The drawing under review shows one solid part. Ordinate dimensions are in mm from its lowest x, y, z. Coordinates: 2 decimals unless noted, no trailing zeros. Loops run counter-clockwise (first coordinate to the right, second up) from the corner with the lowest first, then second, coordinate; pieces in that order, holes last. Notation, with made-up numbers: (-16.5, 48.25) - (20.5, 48.25) arc R20 cw to (20.5, 75.25) - close; hole circle Ø6 at (28, -13.5). An arc over 180 degrees is marked (long way). Answer as a JSON object with one key per item and string values. Group by question number.
Item 1: We need section A-A (y = 0.2). Give the boundary of the cut face in (x, z).
Item 2: Clearance check with a flat-ended pin moving along its axis: pin 1 (3 mm diameter, centred on x = 2.5, z = 1.5, fed in from -Y). State where the tip first meets the part, or that it passes through.
Item 3: To check wall thickness, follow line 1 (Z direction, x = 3, y = 0.2); line 2 (Z direction, x = 2.75, y = 0.25); line 3 (X direction, y = 0.1, z = 7). State the ranges of each line that lie inside material, in increasing order.
Item 4: Mouldability with a two-part tool opening along Y and no side actions: class the marked faces 1 and 2 as released by +Y, released by -Y, zero draft, split by the parting line, or undercut.
Item 5: We need section C-C (x = 2.25). Give the boundary of the cut face in (y, z), then the cut area to 3 significant figures.
Item 6: We need section B-B (z = 7). Give the boundary of the cut face in (x, y).
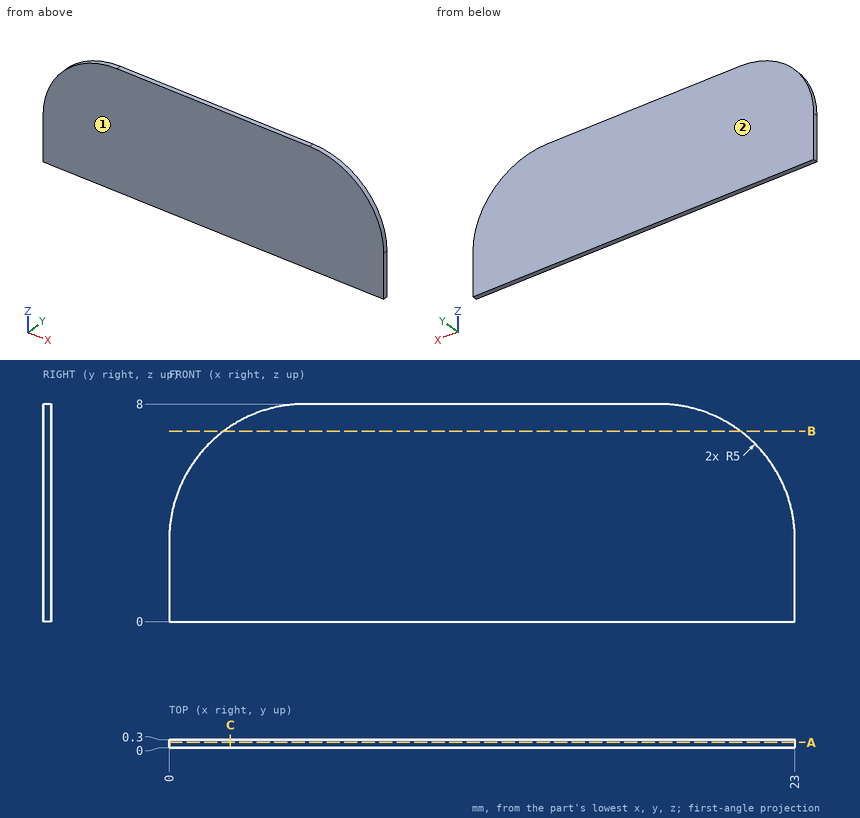
Check sheet entries:
{
 "1": {"outline": "(0, 0) - (23, 0) - (23, 3) arc R5 ccw to (18, 8) - (5, 8) arc R5 ccw to (0, 3) - close"},
 "2": {"pin 1": "stops at y = 0"},
 "3": {"line 1": "z = 0 to 7.58", "line 2": "z = 0 to 7.47", "line 3": "x = 2 to 21"},
 "4": {"face 1": "released by -Y", "face 2": "released by +Y"},
 "5": {"outline": "(0, 0) - (0.3, 0) - (0.3, 7.18) - (0, 7.18) - close", "area": "2.15 mm2"},
 "6": {"outline": "(2, 0) - (21, 0) - (21, 0.3) - (2, 0.3) - close"}
}
